from build123d import *

# Parameters (mm, degrees)
SKETCH_1_R          = 1.625
SKETCH_1_R_2        = 1.575
EXTRUDE_1_DEPTH     = 5
CHAMFER_1_SIZE      = 0.5
CUT_EXTRUDE_1_DEPTH = 10
FILLET_1_R          = 1.8
CHAMFER_2_SIZE      = 0.5
EXTRUDE_2_DEPTH     = 5


with BuildPart() as part:
    # 草图1 → 凸台-拉伸1 (new body)
    with BuildSketch(Plane(origin=(2.5, 0, 0), x_dir=(0, 0, -1), z_dir=(1, 0, 0))):
        with BuildLine():
            Line((10.174472616, -4.871984543), (39.334317565, -7.47039938))
            ThreePointArc((39.334317565, -7.47039938), (47.425031601, -1.057783404), (41.446954522, 7.359097948))
            Line((41.446954522, 7.359097948), (-1.452294145, 15.793998839))
            ThreePointArc((-1.452294145, 15.793998839), (-2.504982909, 15.943374182), (-3.567581162, 15.980138025))
            Line((-3.567581162, 15.980138025), (-108.190291563, 14.033668994))
            ThreePointArc((-108.190291563, 14.033668994), (-109.968090242, 13.840675264), (-111.68308982, 13.334126973))
            Line((-111.68308982, 13.334126973), (-127.759109434, 6.974045822))
            ThreePointArc((-127.759109434, 6.974045822), (-132.233383985, -1.981957648), (-123.818844483, -7.406407472))
            Line((-123.818844483, -7.406407472), (-115.473023263, -6.075436578))
            ThreePointArc((-115.473023263, -6.075436578), (-114.998738119, -6.011395859), (-114.521932102, -5.970120756))
            Line((-114.521932102, -5.970120756), (-91.311587443, -4.519474215))
            ThreePointArc((-91.311587443, -4.519474215), (-90.999847969, -4.50486974), (-90.687804581, -4.5))
            Line((-90.687804581, -4.5), (-9.797958971, -4.5))
            ThreePointArc((-9.797958971, -4.5), (-6.870258752, -4.938171125), (-4.199125273, -6.214285714))
            ThreePointArc((-4.199125273, -6.214285714), (-0.130653307, -7.498861895), (3.980098301, -6.356793021))
            ThreePointArc((3.980098301, -6.356793021), (6.955899906, -5.107988421), (10.174472616, -4.871984543))
        make_face()
        with Locations(Location((-125, 0, 0), (0, 0, 180))):
            Circle(SKETCH_1_R, mode=Mode.SUBTRACT)
        with Locations(Location((0, 0, 0), (0, 0, 180))):
            Circle(SKETCH_1_R, mode=Mode.SUBTRACT)
        with Locations(Location((-106.5, 5, 0), (0, 0, 180))):
            Circle(SKETCH_1_R_2, mode=Mode.SUBTRACT)
        with Locations(Location((-23.5, 8.5, 0), (0, 0, 180))):
            Circle(SKETCH_1_R_2, mode=Mode.SUBTRACT)
        with Locations(Location((40, 0, 0), (0, 0, 180))):
            Circle(SKETCH_1_R, mode=Mode.SUBTRACT)
        with BuildLine():
            Line((-97.531579662, 6.980715987), (-32.542826067, 8.189809077))
            ThreePointArc((-32.542826067, 8.189809077), (-30.505969245, 6.227357985), (-32.468420338, 4.190501164))
            Line((-32.468420338, 4.190501164), (-97.457173933, 2.981408074))
            ThreePointArc((-97.457173933, 2.981408074), (-99.494030755, 4.943859166), (-97.531579662, 6.980715987))
        make_face(mode=Mode.SUBTRACT)
    extrude(amount=-EXTRUDE_1_DEPTH)

    # 倒角1
    chamfer_1_edges = [part.edges().sort_by_distance(p)[0] for p in [
        (-2.5, -1.057783404, -47.425031601),
        (2.5, -7.498861895, 0.130653307),
        (2.5, -4.938171125, 6.870258752),
        (2.5, -4.5, 50.242881776),
        (-2.5, 11.576548393, -19.997330188),
        (2.5, -4.50486974, 90.999847969),
        (2.5, -5.244797486, 102.916759772),
        (2.5, -6.011395859, 114.998738119),
        (2.5, -6.740922025, 119.645933873),
        (2.5, -1.981957648, 132.233383985),
        (2.5, 10.154086398, 119.721099627),
        (2.5, 13.840675264, 109.968090242),
        (2.5, 15.00690351, 55.878936363),
        (2.5, 15.943374182, 2.504982909),
        (2.5, 11.576548393, -19.997330188),
        (-2.5, 15.943374182, 2.504982909),
        (2.5, -1.057783404, -47.425031601),
        (2.5, -6.171191961, -24.754395091),
        (2.5, -5.107988421, -6.955899906),
        (-2.5, 15.00690351, 55.878936363),
        (-2.5, 13.840675264, 109.968090242),
        (-2.5, 10.154086398, 119.721099627),
        (-2.5, -1.981957648, 132.233383985),
        (-2.5, 0, 123.375),
        (2.5, 0, 123.375),
        (-2.5, -6.740922025, 119.645933873),
        (-2.5, 0, -1.625),
        (2.5, 0, -1.625),
        (-2.5, -6.011395859, 114.998738119),
        (-2.5, -5.244797486, 102.916759772),
        (-2.5, -5.107988421, -6.955899906),
        (-2.5, 4.943859166, 99.494030755),
        (-2.5, 7.585262532, 65.037202864),
        (-2.5, 6.227357985, 30.505969245),
        (-2.5, 3.585954619, 64.962797136),
        (2.5, 4.943859166, 99.494030755),
        (2.5, 3.585954619, 64.962797136),
        (2.5, 6.227357985, 30.505969245),
        (-2.5, -4.50486974, 90.999847969),
        (2.5, 7.585262532, 65.037202864),
        (-2.5, -4.5, 50.242881776),
        (-2.5, 5, 104.925),
        (-2.5, -4.938171125, 6.870258752),
        (2.5, 5, 104.925),
        (-2.5, 8.5, 21.925),
        (2.5, 8.5, 21.925),
        (-2.5, -7.498861895, 0.130653307),
        (-2.5, 0, -41.625),
        (2.5, 0, -41.625),
        (-2.5, -6.171191961, -24.754395091),
    ]]
    chamfer(chamfer_1_edges, length=CHAMFER_1_SIZE)

    # Sketch 3D_1 → 切除-拉伸1 (cut)
    with BuildSketch(Plane(origin=(-2.5, 5.468748942, -29.149920979), x_dir=(0, 0.09600082768489282, 0.9953812541352262), z_dir=(-1, 0, 0))):
        Polygon((0, 0), (36.636192851, 3.601725733), (36.990280632, 0), (0.354087782, -3.601725733), align=None)
    extrude(amount=-CUT_EXTRUDE_1_DEPTH, mode=Mode.SUBTRACT)

    # 圆角1
    fillet_1_edges = [part.edges().sort_by_distance(p)[0] for p in [
        (0, 1.917651385, -28.451699987),
        (0, 5.468748942, -29.149920979),
        (0, 9.019846499, 7.669510948),
        (0, 12.570944056, 6.971289956),
    ]]
    fillet(fillet_1_edges, radius=FILLET_1_R)

    # 倒角2
    chamfer_2_edges = [part.edges().sort_by_distance(p)[0] for p in [
        (-2.5, 3.693200164, -28.800810483),
        (2.5, 3.693200164, -28.800810483),
        (-2.5, 5.468748942, -10.391094519),
        (2.5, 5.468748942, -10.391094519),
        (-2.5, 9.019846499, -11.089315511),
        (2.5, 9.019846499, -11.089315511),
        (-2.5, 10.795395278, 7.320400452),
        (2.5, 10.795395278, 7.320400452),
        (2.5, 2.536667318, -28.036109575),
        (-2.5, 2.536667318, -28.036109575),
        (2.5, 5.05315853, -28.530905046),
        (-2.5, 5.05315853, -28.530905046),
        (2.5, 9.435436911, 7.050495015),
        (-2.5, 9.435436911, 7.050495015),
        (2.5, 11.951928123, 6.555699544),
        (-2.5, 11.951928123, 6.555699544),
    ]]
    chamfer(chamfer_2_edges, length=CHAMFER_2_SIZE)

    # Sketch 3D_2 → 凸台-拉伸2 (add)
    with BuildSketch(Plane(origin=(-2.5, 6.354785771, -31.987998048), x_dir=(0, -0.04894175340151768, 0.9988016343468732), z_dir=(-1, 0, 0))):
        Polygon((0, 0), (12.737020213, 4.501231483), (35.673238201, 9.911480997), (42.944661229, 8.12460219), (37.299631195, 0.841435049), (21.568572182, -2.869244472), (5.067736736, -6.761500685), align=None)
        Polygon((63.094756945, -1.716239027), (130.07937311, -0.635871261), (143.056212123, 0), (141.536284317, 10.812456461), (76.338246536, 9.760903695), (52.568858227, 8.596192404), (48.259357211, 3.036112827), (48.527202079, -2.430056119), align=None)
    extrude(amount=-EXTRUDE_2_DEPTH)


solid = part.part
Could you check a few things on this model? Use its own coordinates, in mm. A direction names the side the tool comes from. Give positions to 0.01 mm unless a question says otherwise; leave off trailing zeros. Order: outer loops, then holes, each group sorted by start corner. A loop starts at its lowest first (then second) coordinate and runs counter-clockwise, first axis right, second up. Notation, with made-up numbers: (59, 65.5) - (116, 65.5) arc R35 ccw to (116, 104.5) - close; hole circle Ø5 at (27.25, 38.25). An arc over 180 degrees is marked (long way). Return JSON: item names as keys, results as strings. Group by question number.
Q1. Which directions (+Z, -Z, +X, -X, +Y, -Y) give clear straight access to the entire face, cutting with the end or side of a thin tool? Please do faces 1 (the face through (0.028, -4.926, 6.91)), 2 (the face through (0.028, 11.518, -20.298)).
Q2. Thinking about a two-plate mould opening in Y: for faces 3 (the face through (-2.365, -1.744, 131.919)), 4 (the face through (-2.5, 4, 44)), 5 (the face through (0.028, -0.071, -41.623)), which applies, pulls with the +Y half, pulls with the -Y half, needs draft (parallel to the pull), parting line crosses it, or undercut?
Q3. Suppose I cut it at B-B, the plane z = 120. Please give me the cut outline in (x, y), and give its area (3 significant figures).
Q4. Suppose I cut it at C-C, the plane z = 30. Please give me the cut outline in (x, y).
Q5. Please list where these lines run through material, in increasing order: line 1 along Y through (x, z) = (0.2, 0) (3 decimals); line 2 along Z through (x, y) = (1.8, -1.25); line 3 along Z through (x, y) = (2.15, 0.75). Write a range as [from, to].
Q6. Suppose I cut it at A-A, the plane y = 0. State how many separate pieces and enclosed holes the cut face has, and give its area (3 significant figures).
Q7. Will these pins go through, and if not, where does the flat tip stop? pin 1 Ø4 at (y, z) = (0, 125) entering from -X (3 decimals); pin 2 Ø1 at (x, z) = (0.5, 66) entering from +Y; pin 3 Ø1 at (x, y) = (1, -4.5) entering from -Z.
Resolved:
{
 "1": {"face 1": "+X, -X, -Y", "face 2": "-Z, +X, -X, +Y"},
 "2": {"face 3": "parting line crosses it", "face 4": "needs draft", "face 5": "undercut"},
 "3": {"outline": "(-2.5, -6.29) - (-2, -6.8) - (2, -6.8) - (2.5, -6.29) - (2.5, 9.51) - (2, 10.04) - (-2, 10.04) - (-2.5, 9.51) - close", "area": "83.7 mm2"},
 "4": {"outline": "(-2.5, -4) - (-2, -4.5) - (2, -4.5) - (2.5, -4) - (2.5, 14.99) - (2, 15.49) - (-2, 15.49) - (-2.5, 14.99) - close"},
 "5": {"line 1": "y = [-7.5, -1.625], [1.625, 15.508]", "line 2": "z = [-47.4, -41.04], [-38.96, -1.04], [1.04, 123.96], [126.04, 132.4]", "line 3": "z = [-47.31, -41.61], [-38.39, -1.61], [1.61, 123.39], [126.61, 132.31]"},
 "6": {"separate pieces": "4", "enclosed holes": "0", "area": "849 mm2"},
 "7": {"pin 1": "stops at x = -2.375", "pin 2": "stops at y = 14.83", "pin 3": "stops at z = -46.34"}
}
